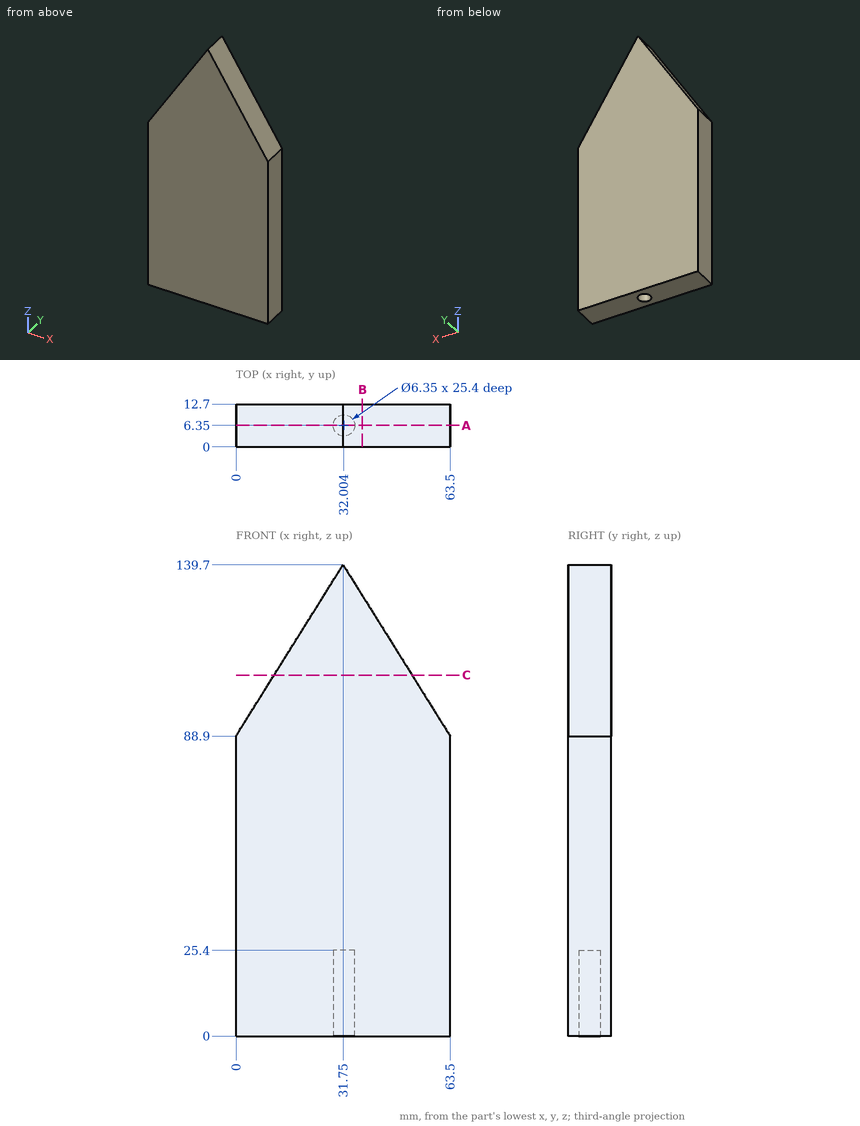
Job drawing, mm, ordinate dimensions from the low corner. One solid piece. Give positions to 0.01 mm unless a question says otherwise; leave off trailing zeros. Order: outer loops, then holes, each group sorted by start corner. A loop starts at its lowest first (then second) coordinate and runs counter-clockwise, first axis right, second up. Notation, with made-up numbers: (55, -2) - (64, -2) arc R34 cw to (64, 28) - close; hole circle Ø8 at (-37, 75.25). An arc over 180 degrees is marked (long way). Answer in a Markdown table with one row per item.
1. Flat gauge pin, fed straight in: pin 1 (1.9 mm diameter, centred on x = 33.5, y = 5.5, fed in from -Z). Where does the tip first touch, or does it go through?
Data:
| item | result |
|---|---|
| pin 1 | stops at z = 25.4 |
2. Probe probe 1 along X at (y, z) = (6.35, 19); probe 2 along Z at (x, y) = (14, 4.75); probe 3 along Z at (x, y) = (47, 9.25). List the from-to ranges inside material, lowest first. Write a range as [from, to].
Data:
| item | result |
|---|---|
| probe 1 | x = [0, 28.83], [35.18, 63.5] |
| probe 2 | z = [0, 111.3] |
| probe 3 | z = [0, 115.3] |
3. Saw through at A-A, the plane y = 6.35. Give the cut face in (x, z), plus the area to 3 significant figures.
Data:
| item | result |
|---|---|
| outline | (0, 0) - (28.83, 0) - (28.83, 25.4) - (35.18, 25.4) - (35.18, 0) - (63.5, 0) - (63.5, 88.9) - (31.75, 139.7) - (0, 88.9) - close |
| area | 7,100 mm² |
4. Saw through at C-C, the plane z = 107. Give the cut face in (x, y), plus the area to 3 significant figures.
Data:
| item | result |
|---|---|
| outline | (11.31, 0) - (52.19, 0) - (52.19, 12.7) - (11.31, 12.7) - close |
| area | 519 mm² |
5. Saw through at B-B, the plane x = 37.5. Give the cut face in (y, z).
Data:
| item | result |
|---|---|
| outline | (0, 0) - (12.7, 0) - (12.7, 130.5) - (0, 130.5) - close |
